Could you check a few things on this drawing? It's one solid part, dimensions in mm from its lowest x, y, z. Round coordinates to 2 decimals unless told otherwise and drop trailing zeros. Order: outer loops, then holes, each group sorted by start corner. A loop starts at its lowest first (then second) coordinate and runs counter-clockwise, first axis right, second up.
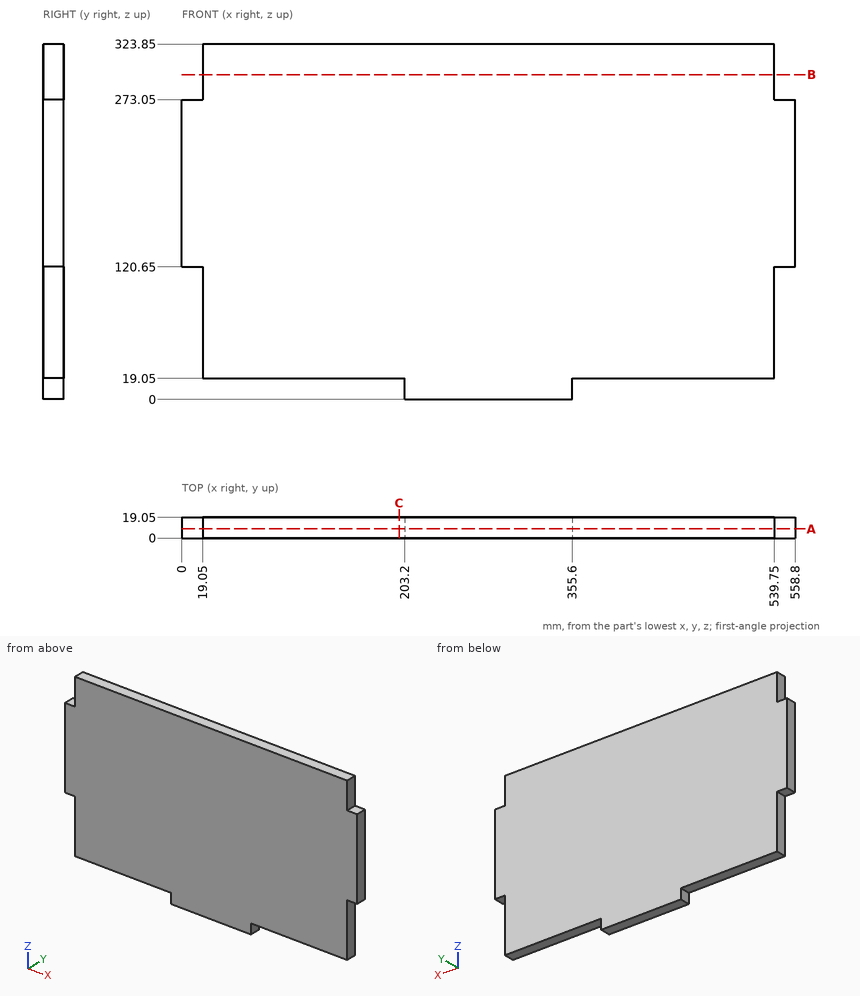
(1) I'm going to push flat-ended pins straight in: pin 1 Ø9.5 at (x, y) = (5, 9.5) entering from +Z; pin 2 Ø4 at (y, z) = (13, 67.5) entering from +X; pin 3 Ø4 at (x, y) = (379.5, 4) entering from -Z. Where does each tip first touch, or does it pass through?
(2) Please list where these lines run through material, in increasing order: probe 1 along Z at (x, y) = (134, 13.75); probe 2 along X at (y, z) = (12.25, 111.5).
(3) I want a section at B-B, the plane z = 296. List the corners of the cut face in (x, y) for me.
(4) I want a section at A-A, the plane y = 8.5. List the corners of the cut face in (x, z) for me.
(5) I want a section at C-C, the plane x = 198. List the corners of the cut face in (y, z) for me.
Ans:
1. pin 1: stops at z = 273.05
1. pin 2: stops at x = 539.75
1. pin 3: stops at z = 19.05
2. probe 1: z = 19.05 to 323.85
2. probe 2: x = 19.05 to 539.75
3. outline: (19.05, 0) - (539.75, 0) - (539.75, 19.05) - (19.05, 19.05) - close
4. outline: (0, 120.65) - (19.05, 120.65) - (19.05, 19.05) - (203.2, 19.05) - (203.2, 0) - (355.6, 0) - (355.6, 19.05) - (539.75, 19.05) - (539.75, 120.65) - (558.8, 120.65) - (558.8, 273.05) - (539.75, 273.05) - (539.75, 323.85) - (19.05, 323.85) - (19.05, 273.05) - (0, 273.05) - close
5. outline: (0, 19.05) - (19.05, 19.05) - (19.05, 323.85) - (0, 323.85) - close
